from build123d import *

# Parameters (mm, degrees)
F0_R     = 6
F1_DEPTH = 15
F2_SIZE  = 0.5


# Not quite as in the source:
# - a feature names something its author has since deleted; it is built from what else it names


with BuildPart() as f1:
    # F0 (on Top) → F1 (new body)
    with BuildSketch(Plane.XY):
        Circle(F0_R)
        Polygon((0.5, 4.8), (0.7508449189, 3.9288970345), (1.7019014352, 3.6198800401), (2.4168607138, 4.1771741991), (3.2258777082, 3.5893889469), (2.9167940342, 2.7372089), (3.5045792865, 1.9281919056), (4.410562781, 1.9588098311), (4.7195797754, 1.0077533149), (3.9686269666, 0.5), (3.9686269666, -0.5), (4.7195797754, -1.0077533149), (4.410562781, -1.9588098311), (3.5045792865, -1.9281919056), (2.9167940342, -2.7372089), (3.2258777082, -3.5893889469), (2.4168607138, -4.1771741991), (1.7019014352, -3.6198800401), (0.7508449189, -3.9288970345), (0.5, -4.8), (-0.5, -4.8), (-0.7508449189, -3.9288970345), (-1.7019014352, -3.6198800401), (-2.4168607138, -4.1771741991), (-3.2258777082, -3.5893889469), (-2.9167940342, -2.7372089), (-3.5045792865, -1.9281919056), (-4.410562781, -1.9588098311), (-4.7195797754, -1.0077533149), (-3.9686269666, -0.5), (-3.9686269666, 0.5), (-4.7195797754, 1.0077533149), (-4.410562781, 1.9588098311), (-3.5045792865, 1.9281919056), (-2.9167940342, 2.7372089), (-3.2258777082, 3.5893889469), (-2.4168607138, 4.1771741991), (-1.7019014352, 3.6198800401), (-0.7508449189, 3.9288970345), (-0.5, 4.8), align=None, mode=Mode.SUBTRACT)
    extrude(amount=F1_DEPTH)

    # F2
    f2_edges = [f1.edges().sort_by_distance(p)[0] for p in [
        (-3.071336, -3.163299, 15),
        (-1.226373, -3.774389, 15),
        (-4.565071, -1.483282, 15),
        (-4.565071, 1.483282, 15),
        (-2.821369, -3.883282, 15),
        (-4.344103, 0.753877, 15),
        (2.821369, 3.883282, 15),
        (-0.625422, -4.364449, 15),
        (-3.210687, -2.3327, 15),
        (-3.071336, 3.163299, 15),
        (1.226373, -3.774389, 15),
        (-4.344103, -0.753877, 15),
        (2.059381, 3.898527, 15),
        (3.071336, -3.163299, 15),
        (4.565071, 1.483282, 15),
        (3.957571, 1.943501, 15),
        (3.968627, 0, 15),
        (3.071336, 3.163299, 15),
        (4.344103, 0.753877, 15),
        (2.821369, -3.883282, 15),
        (3.210687, 2.3327, 15),
        (0.625422, 4.364449, 15),
        (-2.059381, 3.898527, 15),
        (0, 4.8, 15),
        (3.957571, -1.943501, 15),
        (2.059381, -3.898527, 15),
        (-3.210687, 2.3327, 15),
        (-0.625422, 4.364449, 15),
        (0.625422, -4.364449, 15),
        (-2.059381, -3.898527, 15),
        (4.344103, -0.753877, 15),
        (3.210687, -2.3327, 15),
        (0, -4.8, 15),
        (-3.968627, 0, 15),
        (-3.957571, -1.943501, 15),
        (4.565071, -1.483282, 15),
        (-2.821369, 3.883282, 15),
        (1.226373, 3.774389, 15),
        (-3.957571, 1.943501, 15),
        (-1.226373, 3.774389, 15),
        (-2.821369, -3.883282, 0),
        (2.821369, -3.883282, 0),
        (0, -4.8, 0),
        (4.344103, -0.753877, 0),
        (1.226373, -3.774389, 0),
        (-4.344103, 0.753877, 0),
        (2.821369, 3.883282, 0),
        (-0.625422, -4.364449, 0),
        (-3.968627, 0, 0),
        (3.957571, -1.943501, 0),
        (-4.565071, -1.483282, 0),
        (-3.071336, -3.163299, 0),
        (-3.071336, 3.163299, 0),
        (-1.226373, -3.774389, 0),
        (-2.059381, 3.898527, 0),
        (-4.565071, 1.483282, 0),
        (0.625422, 4.364449, 0),
        (3.210687, 2.3327, 0),
        (3.957571, 1.943501, 0),
        (1.226373, 3.774389, 0),
        (-3.210687, 2.3327, 0),
        (3.071336, -3.163299, 0),
        (-1.226373, 3.774389, 0),
        (0.625422, -4.364449, 0),
        (-2.821369, 3.883282, 0),
        (-4.344103, -0.753877, 0),
        (-2.059381, -3.898527, 0),
        (4.344103, 0.753877, 0),
        (-0.625422, 4.364449, 0),
        (-3.210687, -2.3327, 0),
        (-3.957571, 1.943501, 0),
        (4.565071, 1.483282, 0),
        (3.968627, 0, 0),
        (2.059381, 3.898527, 0),
        (2.059381, -3.898527, 0),
        (3.210687, -2.3327, 0),
        (0, 4.8, 0),
        (4.565071, -1.483282, 0),
        (3.071336, 3.163299, 0),
        (-3.957571, -1.943501, 0),
    ]]
    chamfer(f2_edges, length=F2_SIZE)


solid = f1.part
Source: CAD feature listing. Evaluate the final solid. Frame: model axes, mm. A direction names the side the tool comes from. Coordinates: 2 decimals unless noted, no trailing zeros. Loops run counter-clockwise (first coordinate to the right, second up) from the corner with the lowest first, then second, coordinate; pieces in that order, holes last. Notation, with made-up numbers: (-1, 47) -> (21, 47) arc R29 ccw to (21, 80) -> close; hole circle Ø3 at (21, 66). An arc over 180 degrees is marked (long way). Answer in a Markdown table with one row per item. Add a question column.
Q1. Section A-A on y = 0. Return the cut outline in (x, z).
Q2. Section C-C on y = -2.25. Return the cut outline in (x, z).
Q3. Ray query, line 1 along X through (y, z) = (-4, 1); line 2 along Y through (x, z) = (-4, 5.75); line 3 along X through (y, z) = (1.75, 8.25). Return the intervals inside material, ascending.
Q4. Pull-direction query (Y, two-part tool) for faces 4 (the face through (-4, 3, 0)), 5 (the face through (-4.8, -1.57, 14.75)); classes: pulls with the +Y half, pulls with the -Y half, needs draft (parallel to the pull), parting line crosses it, or undercut.
Q5. Reachability of faces 1 (the face through (-3.375, 2.443, 14.698)), 2 (the face through (-3.37, -2.45, 0.3)), 3 (the face through (-4.567, 1.477, 7.402)) from +Z, -Z, +X, -X, +Y, -Y: full face, straight path, thin tool, end or side. Return the list, or none.
Q6. Section B-B on x = 0. Return the cut outline in (y, z).
Q7. Contact query for flat-ended pins moving along their axis: pin 1 Ø1.5 at (x, z) = (-3.5, 2) entering from +Y; pin 2 Ø3 at (x, z) = (3.5, 10.5) entering from -Y. Output: stop coordinate, or through.
Computed values:
| question | item | result |
|---|---|---|
| 1 | outline | (-6, 0) -> (-4.47, 0) -> (-3.97, 0.5) -> (-3.97, 14.5) -> (-4.47, 15) -> (-6, 15) -> close; (3.97, 0.5) -> (4.47, 0) -> (6, 0) -> (6, 15) -> (4.47, 15) -> (3.97, 14.5) -> close |
| 2 | outline | (-5.56, 0) -> (-4.84, 0) -> (-4.61, 0.22) -> (-3.66, 0.18) -> (-3.27, 0.5) -> (-3.27, 14.5) -> (-3.66, 14.82) -> (-4.61, 14.78) -> (-4.84, 15) -> (-5.56, 15) -> close; (3.27, 0.5) -> (3.66, 0.18) -> (4.61, 0.22) -> (4.84, 0) -> (5.56, 0) -> (5.56, 15) -> (4.84, 15) -> (4.61, 14.78) -> (3.66, 14.82) -> (3.27, 14.5) -> close |
| 3 | line 1 | x = -4.47 to -2.66, -2.19 to -0.73, 0.73 to 2.19, 2.66 to 4.47 |
| 3 | line 2 | y = -4.47 to -1.94, -0.52 to 0.52, 1.94 to 4.47 |
| 3 | line 3 | x = -5.74 to -4.48, 4.48 to 5.74 |
| 4 | face 4 | needs draft |
| 4 | face 5 | undercut |
| 5 | face 1 | +Z |
| 5 | face 2 | -Z |
| 5 | face 3 | +Z, -Z |
| 6 | outline | (-6, 0) -> (-5.3, 0) -> (-4.8, 0.5) -> (-4.8, 14.5) -> (-5.3, 15) -> (-6, 15) -> close; (4.8, 0.5) -> (5.3, 0) -> (6, 0) -> (6, 15) -> (5.3, 15) -> (4.8, 14.5) -> close |
| 7 | pin 1 | stops at y = 5.33 |
| 7 | pin 2 | stops at y = -5.66 |
